Design review of the part built by this model. Coordinates are the model's own, in mm. A direction names the side the tool comes from. Coordinates: 2 decimals unless noted, no trailing zeros. Write each loop counter-clockwise with the first axis right and the second up, starting at its lowest first coordinate (ties: lowest second). Pieces come first, ordered by that corner, then holes.
Q1. Take a section at C-C, the plane x = 0.35. Write out the cut boundary in (y, z) (3 decimals).
Q2. For faces 4 (the flat face through (0, -7.5, 0)), 5 (the flat face through (0, -1.25, -3)), list the 3-axis set-ups (+Z, -Z, +X, -X, +Y, -Y) from which the entire face can be reached by the end or side of a thin tool; tool diameter is ignored.
Q3. For pin 1 Ø0.7 at (x, z) = (0, -1.5) entering from +Y; pin 2 Ø1.8 at (y, z) = (3.125, 4.375) entering from +X, all flat-tipped, find the tip position at first contact; note any pin that passes through.
Q4. The part is to be moulded in two halves that separate along Z. For faces 1 (the flat face through (0, -4, -7.5)), 2 (the cylindrical face through (0.01, -2.888, 4.57)), 3 (the flat face through (0, 7.5, 4)), say which applies: released by +Z, released by -Z, zero draft, split by the parting line, or undercut.
Q5. Take a section at A-A, the plane z = -2.25. Write out the cut boundary in (x, y), plus the area to 3 significant figures.
Q6. Take a section at B-B, the plane y = 2. Write out the cut boundary in (x, z).
Q7. Take a section at D-D, the plane y = -3.25. Write out the cut boundary in (x, z), plus the area to 3 significant figures.
Q8. For L1, parallel to Y at x = 0.6, z = 3; L2, parallel to Y at x = -0.55, z = 3.25; L3, parallel to Z at x = -0.3, y = -3.25, list the stretches that pass through material, from the lowest coordinate up.
from build123d import *

# Parameters (mm, degrees)
SALIENTE_EXTRUIR1_DEPTH = 0.7
CROQUIS2_R              = 1.5
CORTAR_EXTRUIR1_DEPTH   = 10


with BuildPart() as part:
    # Croquis1 → Saliente-Extruir1 (new, symmetric)
    with BuildSketch(Plane(origin=(0, 0, 0), x_dir=(0, 0, -1), z_dir=(1, 0, 0))):
        Polygon((-7.5, 7.5), (-7.5, -7.5), (7.5, -7.5), (7.5, -1.25), (-1.25, -1.25), (-1.25, 7.5), align=None)
    extrude(amount=SALIENTE_EXTRUIR1_DEPTH, both=True)

    # Croquis2 → Cortar-Extruir1 (cut, symmetric)
    with BuildSketch(Plane(origin=(0.7, 0, 0), x_dir=(0, 0, -1), z_dir=(1, 0, 0))):
        with Locations((-4.375, -4.375)):
            Circle(CROQUIS2_R)
        with Locations((-4.375, 3.125)):
            Circle(CROQUIS2_R)
        with Locations((3.125, -4.375)):
            Circle(CROQUIS2_R)
    extrude(amount=CORTAR_EXTRUIR1_DEPTH, both=True, mode=Mode.SUBTRACT)


solid = part.part
Responses:
1. outline: (-7.5, -7.5) - (-1.25, -7.5) - (-1.25, 1.25) - (7.5, 1.25) - (7.5, 7.5) - (-7.5, 7.5) - close; hole circle Ø3 at (-4.375, -3.125); hole circle Ø3 at (-4.375, 4.375); hole circle Ø3 at (3.125, 4.375)
2. face 4: +Z, -Z, +X, -X, -Y
2. face 5: -Z, +X, -X, +Y
3. pin 1: stops at y = -1.25
3. pin 2: passes through
4. face 1: released by -Z
4. face 2: undercut
4. face 3: zero draft
5. outline: (-0.7, -7.5) - (0.7, -7.5) - (0.7, -5.59) - (-0.7, -5.59) - close; (-0.7, -3.16) - (0.7, -3.16) - (0.7, -1.25) - (-0.7, -1.25) - close
5. area: 5.34 mm2
6. outline: (-0.7, 1.25) - (0.7, 1.25) - (0.7, 3.38) - (-0.7, 3.38) - close; (-0.7, 5.37) - (0.7, 5.37) - (0.7, 7.5) - (-0.7, 7.5) - close
7. outline: (-0.7, -7.5) - (0.7, -7.5) - (0.7, -4.12) - (-0.7, -4.12) - close; (-0.7, -2.13) - (0.7, -2.13) - (0.7, 3.38) - (-0.7, 3.38) - close; (-0.7, 5.37) - (0.7, 5.37) - (0.7, 7.5) - (-0.7, 7.5) - close
7. area: 15.4 mm2
8. L1: y = -7.5 to -4.97, -3.78 to 2.53, 3.72 to 7.5
8. L2: y = -7.5 to -5.37, -3.38 to 2.13, 4.12 to 7.5
8. L3: z = -7.5 to -4.12, -2.13 to 3.38, 5.37 to 7.5
